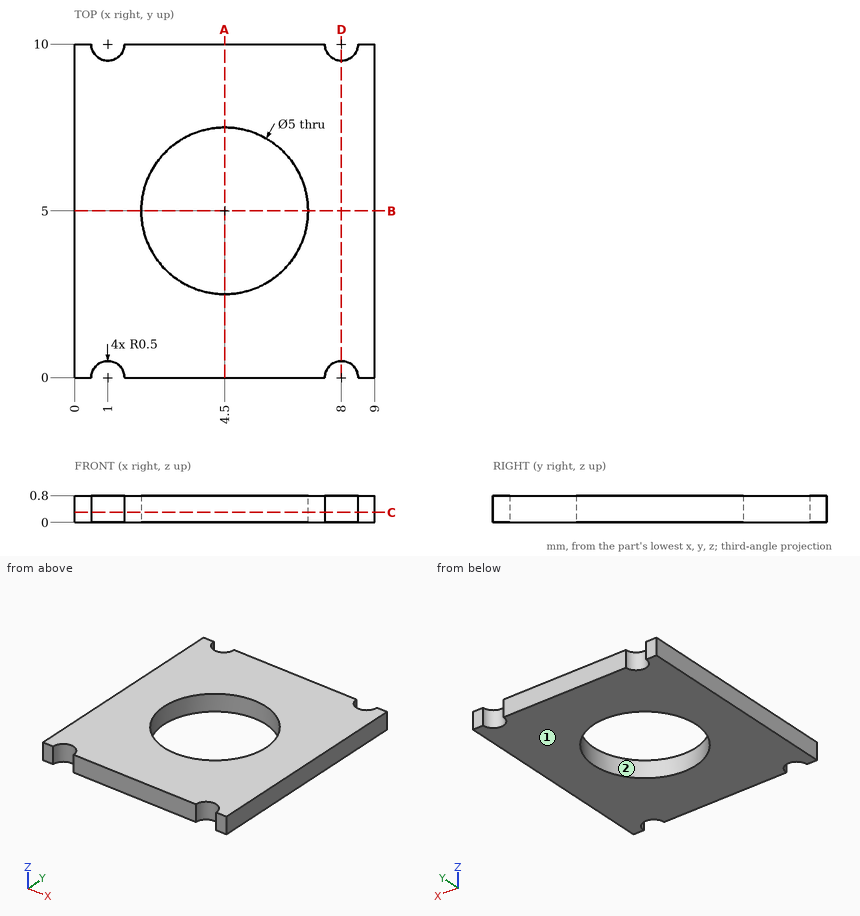
Verification items for this drawing (mm, ordinates from the low corner). Round coordinates to 2 decimals unless told otherwise and drop trailing zeros. Loops run counter-clockwise (first coordinate to the right, second up) from the corner with the lowest first, then second, coordinate; pieces in that order, holes last. Notation, with made-up numbers: (40, 89) -> (88, 89) arc R22 cw to (88, 106) -> close; hole circle Ø4 at (-30, -25). An arc over 180 degrees is marked (long way). Write item = value, one per line. Start each with the question number.
1) Sectioned sample at A-A, the plane x = 4.5. Record the cut outline in (y, z).
2) Release check for a two-part mould opening along X. For the marked faces 1 and 2 record: released by +X, released by -X, zero draft, split by the parting line, or undercut.
3) Thickness scan on probe 1 along Y at (x, z) = (4.5, 0.5); probe 2 along X at (y, z) = (5, 0.35); probe 3 along Y at (x, z) = (5.5, 0.5). Record the ranges inside material, lowest first.
4) Sectioned sample at B-B, the plane y = 5. Record the cut outline in (x, z).
5) Sectioned sample at C-C, the plane z = 0.3. Record the cut outline in (x, y).
6) Sectioned sample at D-D, the plane x = 8. Record the cut outline in (y, z), plus the area to 3 significant figures.
Results are:
q1.outline = (0, 0) -> (2.5, 0) -> (2.5, 0.8) -> (0, 0.8) -> close; (7.5, 0) -> (10, 0) -> (10, 0.8) -> (7.5, 0.8) -> close
q2.face_1 = zero draft
q2.face_2 = undercut
q3.probe_1 = 0 to 2.5, 7.5 to 10
q3.probe_2 = 0 to 2, 7 to 9
q3.probe_3 = 0 to 2.71, 7.29 to 10
q4.outline = (0, 0) -> (2, 0) -> (2, 0.8) -> (0, 0.8) -> close; (7, 0) -> (9, 0) -> (9, 0.8) -> (7, 0.8) -> close
q5.outline = (0, 0) -> (0.5, 0) arc R0.5 cw to (1.5, 0) -> (7.5, 0) arc R0.5 cw to (8.5, 0) -> (9, 0) -> (9, 10) -> (8.5, 10) arc R0.5 cw to (7.5, 10) -> (1.5, 10) arc R0.5 cw to (0.5, 10) -> (0, 10) -> close; hole circle Ø5 at (4.5, 5)
q6.outline = (0.5, 0) -> (9.5, 0) -> (9.5, 0.8) -> (0.5, 0.8) -> close
q6.area = 7.20 mm^2
